Job drawing, mm, ordinate dimensions from the low corner. One solid piece. A direction names the side the tool comes from. Give positions to 0.01 mm unless a question says otherwise; leave off trailing zeros. Loops run counter-clockwise (first coordinate to the right, second up) from the corner with the lowest first, then second, coordinate; pieces in that order, holes last. Notation, with made-up numbers: M -6,82 L 20,82 A23 cw 20,94 Z; hole C -26.75,-24 d1. An arc over 180 degrees is marked long. Put each result on its own line as item: value.
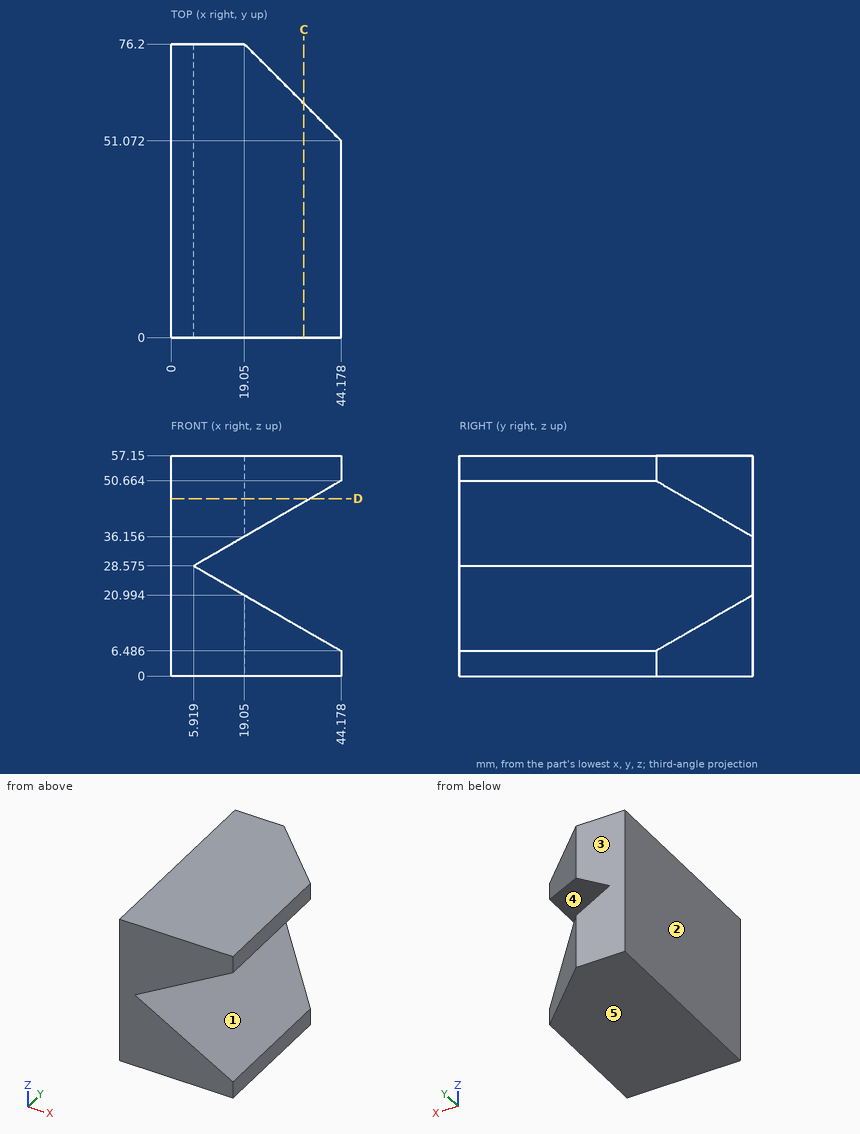
Q1. Probe line 1 (Z direction, x = 10.5, y = 55); line 2 (Z direction, x = 13.5, y = 24); line 3 (X direction, y = 14, z = 29) (1 decimal). List the from-to ranges inside material, lowest first. Write a range as from..to.
Here are the results:
line 1: 0..25.93, 31.22..57.15
line 2: 0..24.2, 32.95..57.15
line 3: 0..6.7
Q2. Mould opens along Z. For the marked faces 3, 4 and 5 say: pulls with the +Z half, pulls with the -Z half, needs draft (parallel to the pull), parting line crosses it, or undercut.
Here are the results:
face 3: needs draft
face 4: undercut
face 5: pulls with the -Z half
Q3. Slice it at D-D (z = 46). List the corners of the cut face in (x, y).
Here are the results:
outline: M 0,0 L 36.1,0 L 36.1,59.15 L 19.05,76.2 L 0,76.2 Z
Q4. Tool access for the marked faces 1 and 2: list every direction of +Z, -Z, +X, -X, +Y, -Y with a clear straight run to the whole face (end or side of a thin tool).
Here are the results:
face 1: +X, +Y, -Y
face 2: +Z, -Z, -X, +Y, -Y
Q5. Slice it at C-C (x = 34.5). List the corners of the cut face in (y, z), and give its area (3 significant figures).
Here are the results:
outline: M 0,0 L 60.75,0 L 60.75,12.07 L 0,12.07 Z; M 0,45.08 L 60.75,45.08 L 60.75,57.15 L 0,57.15 Z
area: 1,470 mm²
